Answer from the drawing. Dimensions are ordinates in mm from the lowest x, y and z of the part. A direction names the side the tool comes from. Round coordinates to 2 decimals unless told otherwise and drop trailing zeros. Loops run counter-clockwise (first coordinate to the right, second up) from the corner with the lowest first, then second, coordinate; pieces in that order, holes last.
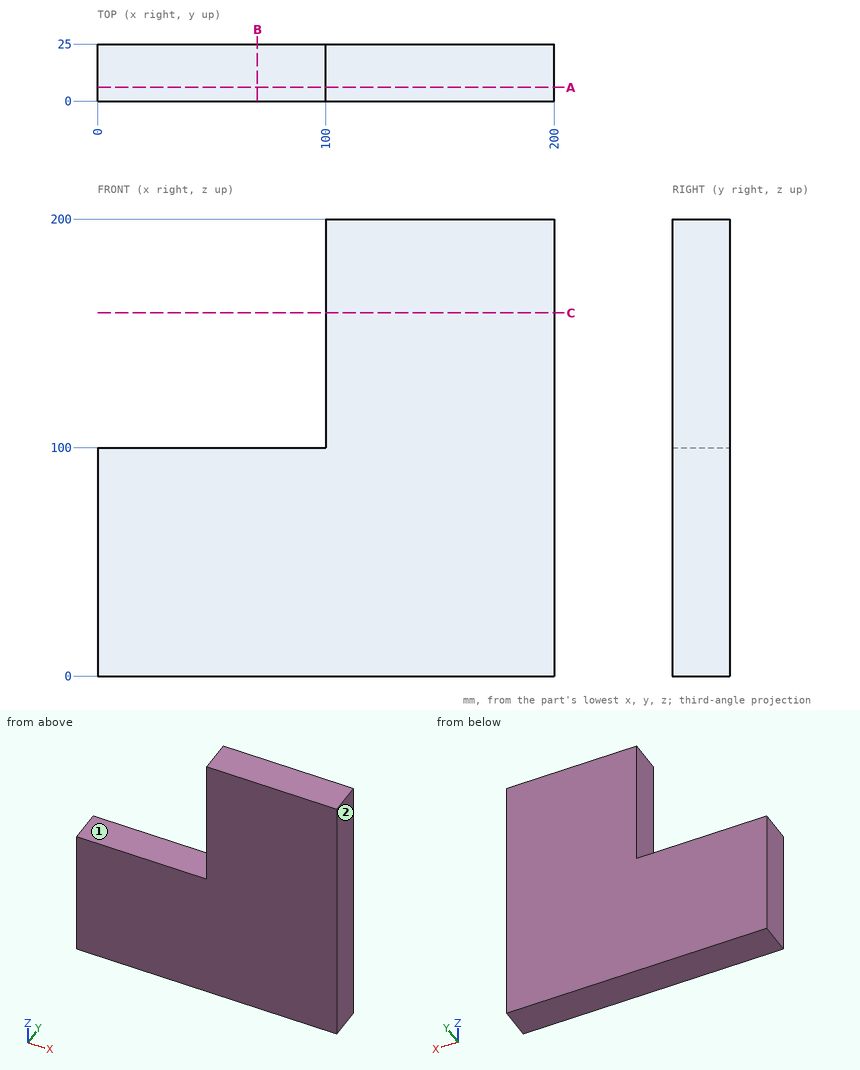
Item 1: Section B-B, the plane x = 70 is taken. Give the vertices of the cut face in (y, z).
Item 2: Section A-A, the plane y = 6 is taken. Give the vertices of the cut face in (x, z).
Item 3: For the marked faces 1 and 2, determine the directions among +Z, -Z, +X, -X, +Y, -Y from which every point of the face is accessible in a straight line to the end or side of a thin tool.
Item 4: Each of these flat-tipped pins is pushed along its axis until it touches: P1, Ø8, axis at x = 47, z = 50.5, coming from the -Y side; P2, Ø8, axis at y = 20.5, z = 125.5, coming from the -X side. Where does it stop, or does it pass through?
Item 5: Straight lines are drawn through the part: line 1 (Z direction, x = 71.5, y = 3); line 2 (X direction, y = 13.75, z = 189). For each, find the intervals that lie inside material, in ascending order.
Item 6: Section C-C, the plane z = 159 is taken. Give the vertices of the cut face in (x, y).
Answer below:
1. outline: (0, 0) - (25, 0) - (25, 100) - (0, 100) - close
2. outline: (0, 0) - (200, 0) - (200, 200) - (100, 200) - (100, 100) - (0, 100) - close
3. face 1: +Z, -X, +Y, -Y
3. face 2: +Z, -Z, +X, +Y, -Y
4. P1: stops at y = 0
4. P2: stops at x = 100
5. line 1: z = 0 to 100
5. line 2: x = 100 to 200
6. outline: (100, 0) - (200, 0) - (200, 25) - (100, 25) - close
